Geometry: final body of the model. Coordinates: model frame, mm. Face numbers are marked on the shaded views. A direction names the side the tool comes from. Give positions to 0.01 mm unless a question says otherwise; leave off trailing zeros. Loops run counter-clockwise (first coordinate to the right, second up) from the corner with the lowest first, then second, coordinate; pieces in that order, holes last. Notation, with made-up numbers: (-7, 38.5) - (45, 38.5) arc R25 ccw to (45, 76.5) - close; hole circle Ø11 at (13, -35.75). An arc over 180 degrees is marked (long way). Use one line per item in the form item = value.
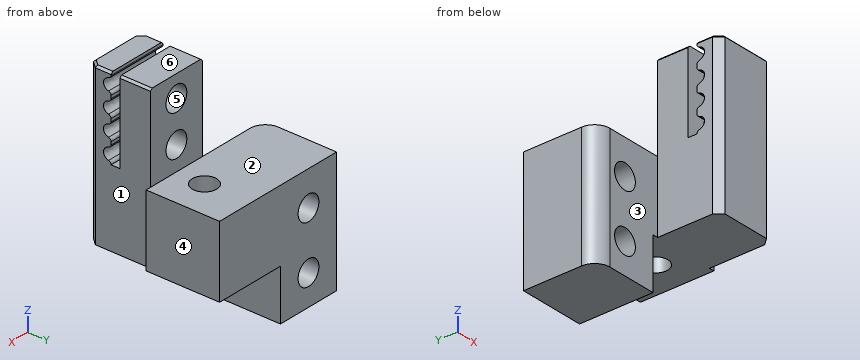
```python
from build123d import *

# Parameters (mm, degrees)
BOSS_EXTRUDE1_DEPTH     = 13
SKETCH6_W               = 6
SKETCH6_H               = 5
BOSS_EXTRUDE4_DEPTH     = 5.6
SKETCH16_W              = 6
SKETCH16_H              = 8
BOSS_EXTRUDE5_DEPTH     = 0.1
CUT_EXTRUDE6_DEPTH      = 4
CUT_EXTRUDE6_DEPTH_BACK = 3.6
SKETCH15_R              = 1.2
CUT_EXTRUDE7_DEPTH      = 8.7202
CUT_EXTRUDE8_START      = -0.2202
SKETCH19_W              = 6
SKETCH19_H              = 8
SKETCH19_R              = 1.2
CUT_EXTRUDE8_DEPTH      = 0.2202
SKETCH12_R              = 1.2
CUT_EXTRUDE5_DEPTH      = 6
SKETCH21_R              = 1.2
BOSS_EXTRUDE6_DEPTH     = 2.5
SKETCH24_W              = 6
SKETCH24_H              = 5.5
CUT_EXTRUDE10_DEPTH     = 8.5
BOSS_EXTRUDE8_DEPTH     = 7.2
FILLET4_R               = 1.5
SKETCH26_R              = 1.2
CUT_EXTRUDE11_DEPTH     = 10
CHAMFER1_SIZE           = 0.2
BOSS_EXTRUDE9_DEPTH     = 5
SKETCH31_R              = 1.2
CUT_EXTRUDE12_DEPTH     = 8


with BuildPart() as part:
    # Sketch1 → Boss-Extrude1 (new body)
    with BuildSketch(Plane.XY):
        Polygon((3, 3.05), (3, -2.253801214), (2.388188946, -2.95), (-2.388188946, -2.95), (-3, -2.253801214), (-3, 3.05), align=None)
    extrude(amount=BOSS_EXTRUDE1_DEPTH)

    # Sketch6 → Boss-Extrude4 (add)
    with BuildSketch(Plane(origin=(0, 3.05, 0), x_dir=(1, 0, 0), z_dir=(0, 1, 0))):
        with Locations((0, -2.5)):
            Rectangle(SKETCH6_W, SKETCH6_H)
    extrude(amount=BOSS_EXTRUDE4_DEPTH)

    # Sketch16 → Boss-Extrude5 (add)
    with BuildSketch(Plane(origin=(0, 3.05, 0), x_dir=(1, 0, 0), z_dir=(0, 1, 0))):
        with Locations((0, -9)):
            Rectangle(SKETCH16_W, SKETCH16_H)
    extrude(amount=BOSS_EXTRUDE5_DEPTH)

    # Sketch18 → Cut-Extrude6 (cut, two sides: drawn at the far end of the back side and taken through both)
    with BuildSketch(Plane(origin=(0, 0, 0), x_dir=(0, 0, -1), z_dir=(1, 0, 0)).offset(-CUT_EXTRUDE6_DEPTH_BACK)):
        with BuildLine():
            Line((-8.8572, -0.0702), (-12.8572, -0.0702))
            Line((-12.8572, -0.0702), (-13, -0.0702))
            Line((-13, -0.0702), (-13, -0.7))
            Line((-13, -0.7), (-12.8572, -0.7))
            Line((-12.8572, -0.7), (-12.7144, -0.7))
            add(Edge.make_bspline(
                [(-12.7144, -0.7), (-12.5198, -0.7), (-12.43, -0.9509)],
                knots=[0.103448276, 0.103448276, 0.103448276, 0.137931034, 0.137931034, 0.137931034], degree=2))
            add(Edge.make_bspline(
                [(-12.43, -0.9509), (-12.3594, -1.2388), (-12.13, -1.45), (-11.8572, -1.45)],
                knots=[0.137931034, 0.137931034, 0.137931034, 0.137931034, 0.172413793, 0.172413793, 0.172413793, 0.172413793], degree=3))
            add(Edge.make_bspline(
                [(-11.8572, -1.45), (-11.5844, -1.45), (-11.355, -1.2388), (-11.2844, -0.9509)],
                knots=[0.172413793, 0.172413793, 0.172413793, 0.172413793, 0.206896552, 0.206896552, 0.206896552, 0.206896552], degree=3))
            add(Edge.make_bspline(
                [(-11.2844, -0.9509), (-11.1946, -0.7), (-11, -0.7)],
                knots=[0.206896552, 0.206896552, 0.206896552, 0.24137931, 0.24137931, 0.24137931], degree=2))
            Line((-11, -0.7), (-10.8572, -0.7))
            Line((-10.8572, -0.7), (-10.7144, -0.7))
            add(Edge.make_bspline(
                [(-10.7144, -0.7), (-10.5198, -0.7), (-10.43, -0.9509)],
                knots=[0.310344828, 0.310344828, 0.310344828, 0.344827586, 0.344827586, 0.344827586], degree=2))
            add(Edge.make_bspline(
                [(-10.43, -0.9509), (-10.3594, -1.2388), (-10.13, -1.45), (-9.8572, -1.45)],
                knots=[0.344827586, 0.344827586, 0.344827586, 0.344827586, 0.379310345, 0.379310345, 0.379310345, 0.379310345], degree=3))
            add(Edge.make_bspline(
                [(-9.8572, -1.45), (-9.5844, -1.45), (-9.355, -1.2388), (-9.2844, -0.9509)],
                knots=[0.379310345, 0.379310345, 0.379310345, 0.379310345, 0.413793103, 0.413793103, 0.413793103, 0.413793103], degree=3))
            add(Edge.make_bspline(
                [(-9.2844, -0.9509), (-9.1946, -0.7), (-9, -0.7)],
                knots=[0.413793103, 0.413793103, 0.413793103, 0.448275862, 0.448275862, 0.448275862], degree=2))
            Line((-9, -0.7), (-8.8572, -0.7))
            Line((-8.8572, -0.7), (-8.7144, -0.7))
            add(Edge.make_bspline(
                [(-8.7144, -0.7), (-8.5198, -0.7), (-8.43, -0.9509)],
                knots=[0.517241379, 0.517241379, 0.517241379, 0.551724138, 0.551724138, 0.551724138], degree=2))
            add(Edge.make_bspline(
                [(-8.43, -0.9509), (-8.3594, -1.2388), (-8.13, -1.45), (-7.8572, -1.45)],
                knots=[0.551724138, 0.551724138, 0.551724138, 0.551724138, 0.586206897, 0.586206897, 0.586206897, 0.586206897], degree=3))
            add(Edge.make_bspline(
                [(-7.8572, -1.45), (-7.5844, -1.45), (-7.355, -1.2388), (-7.2844, -0.9509)],
                knots=[0.586206897, 0.586206897, 0.586206897, 0.586206897, 0.620689655, 0.620689655, 0.620689655, 0.620689655], degree=3))
            add(Edge.make_bspline(
                [(-7.2844, -0.9509), (-7.1946, -0.7), (-7, -0.7)],
                knots=[0.620689655, 0.620689655, 0.620689655, 0.655172414, 0.655172414, 0.655172414], degree=2))
            Line((-7, -0.7), (-6.8572, -0.7))
            Line((-6.8572, -0.7), (-6.7144, -0.7))
            add(Edge.make_bspline(
                [(-6.7144, -0.7), (-6.5198, -0.7), (-6.43, -0.9509)],
                knots=[0.724137931, 0.724137931, 0.724137931, 0.75862069, 0.75862069, 0.75862069], degree=2))
            add(Edge.make_bspline(
                [(-6.43, -0.9509), (-6.3594, -1.2388), (-6.13, -1.45), (-5.8572, -1.45)],
                knots=[0.75862069, 0.75862069, 0.75862069, 0.75862069, 0.793103448, 0.793103448, 0.793103448, 0.793103448], degree=3))
            add(Edge.make_bspline(
                [(-5.8572, -1.45), (-5.5844, -1.45), (-5.355, -1.2388), (-5.2844, -0.9509)],
                knots=[0.793103448, 0.793103448, 0.793103448, 0.793103448, 0.827586207, 0.827586207, 0.827586207, 0.827586207], degree=3))
            add(Edge.make_bspline(
                [(-5.2844, -0.9509), (-5.1946, -0.7), (-5, -0.7)],
                knots=[0.827586207, 0.827586207, 0.827586207, 0.862068966, 0.862068966, 0.862068966], degree=2))
            Line((-5, -0.7), (-5, -0.0702))
            Line((-5, -0.0702), (-8.8572, -0.0702))
        make_face()
    extrude(amount=CUT_EXTRUDE6_DEPTH + CUT_EXTRUDE6_DEPTH_BACK, mode=Mode.SUBTRACT)

    # Sketch15 → Cut-Extrude7 (cut)
    with BuildSketch(Plane(origin=(0, 8.65, 0), x_dir=(1, 0, 0), z_dir=(0, 1, 0))):
        with Locations(Location((0, -10.8572, 0), (0, 0, 180))):
            Circle(SKETCH15_R)
        with Locations(Location((0, -6.8572, 0), (0, 0, 180))):
            Circle(SKETCH15_R)
    extrude(amount=-CUT_EXTRUDE7_DEPTH, mode=Mode.SUBTRACT)

    # Sketch19 → Cut-Extrude8 (cut)
    with BuildSketch(Plane.XZ.offset(0.0702).offset(CUT_EXTRUDE8_START)):
        with Locations((0, 9)):
            Rectangle(SKETCH19_W, SKETCH19_H)
        with Locations(Location((0, 10.8572, 0), (0, 0, 180))):
            Circle(SKETCH19_R, mode=Mode.SUBTRACT)
        with Locations(Location((0, 6.8572, 0), (0, 0, 180))):
            Circle(SKETCH19_R, mode=Mode.SUBTRACT)
    extrude(amount=CUT_EXTRUDE8_DEPTH, mode=Mode.SUBTRACT)

    # Sketch12 → Cut-Extrude5 (cut)
    with BuildSketch(Plane.XY.offset(5)):
        with Locations((0, 5.85)):
            Circle(SKETCH12_R)
    extrude(amount=-CUT_EXTRUDE5_DEPTH, mode=Mode.SUBTRACT)

    # Sketch21 → Boss-Extrude6 (add)
    with BuildSketch(Plane(origin=(0, 0, 0), x_dir=(-1, 0, 0), z_dir=(0, 0, -1))):
        Polygon((-2.388188946, -2.95), (2.388188946, -2.95), (3, -2.253801214), (3, 8.65), (-3, 8.65), (-3, -2.253801214), align=None)
        with Locations(Location((0, 5.85, 0), (0, 0, 180))):
            Circle(SKETCH21_R, mode=Mode.SUBTRACT)
    extrude(amount=BOSS_EXTRUDE6_DEPTH)

    # Sketch24 → Cut-Extrude10 (cut)
    with BuildSketch(Plane.XY.offset(5)):
        with Locations((0, 5.9)):
            Rectangle(SKETCH24_W, SKETCH24_H)
    extrude(amount=-CUT_EXTRUDE10_DEPTH, mode=Mode.SUBTRACT)

    # Sketch25 → Boss-Extrude8 (add)
    with BuildSketch(Plane(origin=(0, 3.15, 0), x_dir=(1, 0, 0), z_dir=(0, 1, 0))):
        Polygon((-10, -4.5), (0, -4.5), (3.5, -4.5), (3.5, 2.5), (-10, 2.5), align=None)
    extrude(amount=BOSS_EXTRUDE8_DEPTH)

    # Fillet4
    fillet4_edges = [part.edges().sort_by_distance(p)[0] for p in [
        (-10, 3.15, 1),
    ]]
    fillet(fillet4_edges, radius=FILLET4_R)

    # Sketch26 → Cut-Extrude11 (cut)
    with BuildSketch(Plane.XY.offset(4.5)):
        with Locations((0, 5.9)):
            Circle(SKETCH26_R)
    extrude(amount=-CUT_EXTRUDE11_DEPTH, mode=Mode.SUBTRACT)

    # Chamfer1
    chamfer1_edges = [part.edges().sort_by_distance(p)[0] for p in [
        (-2.694094473, -2.601900607, 13),
        (0, -2.95, 13),
        (2.694094473, -2.601900607, 13),
        (3, 1.65, 13),
        (3, -1.476900607, 13),
        (-3, -1.476900607, 13),
        (-3, 1.65, 13),
    ]]
    chamfer(chamfer1_edges, length=CHAMFER1_SIZE)

    # Sketch29 → Boss-Extrude9 (add)
    with BuildSketch(Plane(origin=(0, 0, -2.5), x_dir=(-1, 0, 0), z_dir=(0, 0, -1))):
        with BuildLine():
            Line((3.53, 3.15), (3.53, 10.35))
            Line((3.53, 10.35), (10, 10.35))
            Line((10, 10.35), (10, 4.65))
            ThreePointArc((10, 4.65), (9.560660172, 3.589339828), (8.5, 3.15))
            Line((8.5, 3.15), (3.53, 3.15))
        make_face()
    extrude(amount=BOSS_EXTRUDE9_DEPTH)

    # Sketch31 → Cut-Extrude12 (cut)
    with BuildSketch(Plane(origin=(0, 10.35, 0), x_dir=(1, 0, 0), z_dir=(0, 1, 0))):
        with Locations(Location((-6.765, 4.5, 0), (0, 0, 180))):
            Circle(SKETCH31_R)
        with Locations(Location((-6.765, -1.1, 0), (0, 0, 180))):
            Circle(SKETCH31_R)
    extrude(amount=-CUT_EXTRUDE12_DEPTH, mode=Mode.SUBTRACT)


solid = part.part
```
(1) Cut plane C-C (x = -6.75). Return the cut outline in (y, z).
Solution:
outline = (3.15, -7.5) - (10.35, -7.5) - (10.35, -5.7) - (3.15, -5.7) - close; (3.15, -3.3) - (10.35, -3.3) - (10.35, -0.1) - (3.15, -0.1) - close; (3.15, 2.3) - (10.35, 2.3) - (10.35, 4.5) - (3.15, 4.5) - close
(2) Cut plane B-B (y = 5.9). Return the cut outline in (x, z) (3 decimals).
Solution:
outline = (-10, -7.5) - (-3.53, -7.5) - (-3.53, -2.5) - (-1.2, -2.5) - (-1.2, 4.5) - (-10, 4.5) - close; (1.2, -2.5) - (3.5, -2.5) - (3.5, 4.5) - (1.2, 4.5) - close; hole circle Ø2.4 at (-6.765, -4.5); hole circle Ø2.4 at (-6.765, 1.1)
(3) Pin query (flat end, axial travel): P1, Ø3, axis at x = 0, y = 5.9, coming from the -Z side; P2, Ø4.5, axis at x = -6, z = 1, coming from the -Y side; P3, Ø6, axis at y = 1.5, z = 0.5, coming from the -X side. Return the tip coordinate at first contact, or that it passes through.
Solution:
P1 = -2.5
P2 = 3.15
P3 = -9.99
(4) Cut plane A-A (z = 1.1). Return the cut outline in (x, y) (3 decimals), plus the area to 3 significant figures.
Solution:
outline = (-10, 4.65) arc R1.5 ccw to (-8.5, 3.15) - (-7.965, 3.15) - (-7.965, 10.35) - (-10, 10.35) - close; (-5.565, 3.15) - (-3, 3.15) - (-3, -2.254) - (-2.388, -2.95) - (2.388, -2.95) - (3, -2.254) - (3, 3.15) - (3.5, 3.15) - (3.5, 10.35) - (-5.565, 10.35) - close; hole circle Ø2.4 at (0, 5.9)
area = 111 mm2
(5) Pull-direction query (X, two-part tool) for the marked faces 4, 5 and 6; classes: released by +X, released by -X, zero draft, split by the parting line, or undercut.
Solution:
face_4 = released by +X
face_5 = undercut
face_6 = zero draft
(6) Access query for the marked faces 1, 2 and 3. Directions: +Z, -Z, +X, -X, +Y, -Y. A direction counts if a zero-diameter tool reaches every point of the face in a straight line with its end or side. Return the directions, or none.
Solution:
face_1 = +Z, -Z, +X, -Y
face_2 = +Z, +X, -X, +Y
face_3 = +Z, -Z, -X, -Y
(7) Material intervals for L1, parallel to Z at x = 0, y = 2.55; L2, parallel to Z at x = -1, y = 3; L3, parallel to X at y = 3, z = 6.75, sorted ascending. Write a range as from..to.
Solution:
L1 = -2.5..5.66, 8.06..9.66, 12.06..13
L2 = -2.5..6.19, 7.52..10.19, 11.52..13
L3 = -3..-1.2, 1.2..3
(8) Cut plane D-D (z = -2). Return the cut outline in (x, y), plus the area to 3 significant figures.
Solution:
outline = (-10, 4.65) arc R1.5 ccw to (-8.5, 3.15) - (-3, 3.15) - (-3, -2.25) - (-2.39, -2.95) - (2.39, -2.95) - (3, -2.25) - (3, 3.15) - (3.5, 3.15) - (3.5, 10.35) - (-10, 10.35) - close; hole circle Ø2.4 at (0, 5.9)
area = 128 mm2
